Work out the finished part from the listing and answer in its coordinate system (mm). Round coordinates to 2 decimals unless told otherwise and drop trailing zeros. Write each loop counter-clockwise with the first axis right and the second up, starting at its lowest first coordinate (ties: lowest second). Pieces come first, ordered by that corner, then holes. Notation, with made-up numbers: M 53,-39.5 L 83,-39.5 A23 cw 83,-3.5 Z; hole C 57,59.5 d11. An arc over 180 degrees is marked long. One line per item, written item: value. Start each with the question number.
Q1. Given pin 1 Ø3 at (y, z) = (2.5, 8.5) entering from +X; pin 2 Ø3 at (y, z) = (-0.5, 25.5) entering from +X; pin 3 Ø1 at (x, z) = (-2.5, 23.5) entering from +Y, each flat-ended and moving along its own axis, determine where each tip first touches the part or whether it passes through.
Q2. Find section A-A (x = 0). Write down the section's boundary in (y, z), and give its area (3 significant figures).
Q3. Consider probe 1 along Y at (x, z) = (-0.5, 24.75); probe 2 along Y at (x, z) = (-1, 19.5); probe 3 along X at (y, z) = (-1.5, 20.5). Determine where each line is inside the solid, lowest interval first.
Q4. Find section D-D (y = -2). Write down the section's boundary in (x, z).
Q5. Find section B-B (y = 0). Write down the section's boundary in (x, z).
Q6. Find section C-C (z = 8.25). Write down the section's boundary in (x, y).
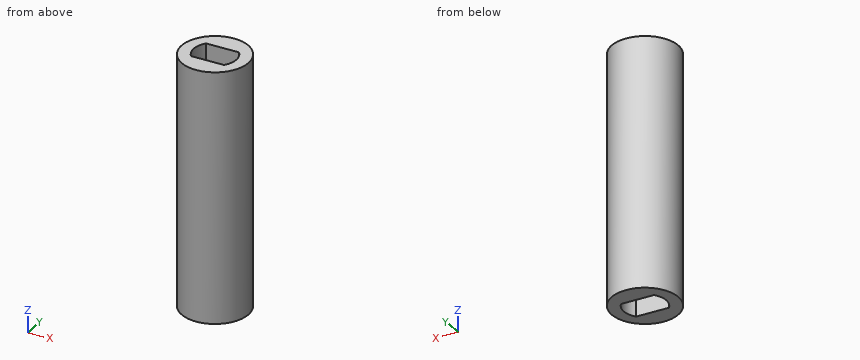
Autodesk Fusion 360 part; units mm, degrees
sketch "Sketch1" plane through (0, 0, 0) normal (0, 0, 1) x (1, 0, 0)
  circle A0 centre (0, 0) radius 4
  line L0 (0, 0) -> (0, 1.6)
  line L1 (0, 0) -> (0, -1.6)
  line L2 (-1.9879, 1.5971) -> (1.9879, 1.5971)
  line L3 (-1.9878, -1.5972) -> (1.9878, -1.5972)
  arc A1 (-1.9879, 1.5971) -> (-1.9878, -1.5972) centre (0, 0) ccw
  arc A2 (1.9878, -1.5972) -> (1.9879, 1.5971) centre (0, 0) ccw
  dimension "d1" = 8
  dimension "d2" = 5.1
  dimension "d3" = 1.6
  dimension "d4" = 1.6
extrude "Extrude1" add sketch "Sketch1" along normal blind 30
The answers:
1. pin 1: x = 3.87
1. pin 2: x = 4
1. pin 3: y = 3.46
2. outline: M -4,0 L -1.6,0 L -1.6,30 L -4,30 Z; M 1.6,0 L 4,0 L 4,30 L 1.6,30 Z
2. area: 144 mm2
3. probe 1: -3.97 to -1.6, 1.6 to 3.97
3. probe 2: -3.87 to -1.6, 1.6 to 3.87
3. probe 3: -3.71 to -2.06, 2.06 to 3.71
4. outline: M -3.46,0 L 3.46,0 L 3.46,30 L -3.46,30 Z
5. outline: M -4,0 L -2.55,0 L -2.55,30 L -4,30 Z; M 2.55,0 L 4,0 L 4,30 L 2.55,30 Z
6. outline: C 0,0 d8; hole M -1.99,-1.6 L 1.99,-1.6 A2.55 ccw 1.99,1.6 L -1.99,1.6 A2.55 ccw Z
